Input: part model. Units: mm. Frame: model coordinates. A direction names the side the tool comes from. Coordinates: 2 decimals unless noted, no trailing zeros. Write each loop counter-clockwise with the first axis right and the second up, starting at its lowest first coordinate (ties: lowest second). Pieces come first, ordered by that corner, then holes. Notation, with made-up numbers: M -19,84 L 14,84 A32 ccw 14,114 Z; hole C 37,83.5 d9. An arc over 180 degrees is marked long. Write each question's results on one line, items separated by ' | '. Start each with the question number.
1. First-contact query: pin 1 (4.5 mm diameter, centred on x = 36.5, z = -2.5, fed in from +Y); pin 2 (1.5 mm diameter, centred on x = 38, z = 2.5, fed in from -Y); pin 3 (4 mm diameter, centred on y = 17.5, z = 2, fed in from -X). Flat tips, straight axial feed; report the tip coordinate or a pass-through.
2. Section query B-B, the plane z = -1.5. Output: boundary loops of the cut face in (x, y), and give its area (3 significant figures).
3. Set-up query: faces 5 (the flat face through (36, 20, -3)), 6 (the flat face through (38, 18.6, -2.5)), 7 (the cylindrical face through (17.94, 31.46, 4.81)). Return all of +Z, -Z, +X, -X, +Y, -Y with unobstructed straight access to the full face (end or side cutting, diameter ignored); none if empty.
4. Section query A-A, the plane x = -7. Output: boundary loops of the cut face in (y, z).
5. Section query C-C, the plane x = 1.5. Output: boundary loops of the cut face in (y, z).
6. Ray query, probe 1 along Y at (x, z) = (37.5, -2); probe 2 along Y at (x, z) = (-5, 0.75); probe 3 along X at (y, z) = (25, 3.5). Return the intervals inside material, ascending.
7. Section query D-D, the plane y = 5.5. Output: boundary loops of the cut face in (x, z).
8. Pull-direction query (Y, two-part tool) for faces 1 (the flat face through (10, 29, 2)), 2 (the flat face through (18.9, 30.2, 0.6)), 3 (the flat face through (39, 0, 2)), 4 (the flat face through (31, 15, 5)); classes: +Y half, -Y half, draft (parallel to the pull), parting line (faces both ways), or undercut.
```python
from build123d import *

# Parameters (mm, degrees)
SKETCH1_W           = 73
SKETCH1_H           = 29
BOSS_EXTRUDE1_DEPTH = 5
SKETCH2_R           = 1
CUT_EXTRUDE1_DEPTH  = 35
SKETCH3_W           = 4
SKETCH3_H           = 6
BOSS_EXTRUDE2_DEPTH = 5
SKETCH4_W           = 3
SKETCH4_H           = 2
CUT_EXTRUDE2_DEPTH  = 10
SKETCH5_R           = 2.5
BOSS_EXTRUDE3_DEPTH = 5
CUT_EXTRUDE3_DEPTH  = 25
FILLET1_R           = 1


with BuildPart() as part:
    # Sketch1 → Boss-Extrude1 (new body)
    with BuildSketch(Plane.XY):
        with Locations((36.5, 14.5)):
            Rectangle(SKETCH1_W, SKETCH1_H)
        Polygon((-10, 29), (0, 29), (5, 29), (5, 33), (-10, 33), align=None)
        Polygon((5, 0), (0, 0), (-10, 0), (-10, -4), (5, -4), align=None)
    extrude(amount=BOSS_EXTRUDE1_DEPTH)

    # Sketch2 → Cut-Extrude1 (cut)
    with BuildSketch(Plane(origin=(0, 33, 0), x_dir=(1, 0, 0), z_dir=(0, 1, 0))):
        with Locations(Location((-7, -2.46940408, 0), (0, 0, 270))):
            Circle(SKETCH2_R)
    extrude(amount=-CUT_EXTRUDE1_DEPTH, mode=Mode.SUBTRACT)

    # Sketch3 → Boss-Extrude2 (add)
    with BuildSketch(Plane(origin=(0, 0, 0), x_dir=(-1, 0, 0), z_dir=(0, 0, -1))):
        with Locations((-36, 20)):
            Rectangle(SKETCH3_W, SKETCH3_H)
    extrude(amount=BOSS_EXTRUDE2_DEPTH)

    # Sketch4 → Cut-Extrude2 (cut)
    with BuildSketch(Plane(origin=(38, 0, 0), x_dir=(0, 0, -1), z_dir=(1, 0, 0))):
        with Locations((1.5, 20)):
            Rectangle(SKETCH4_W, SKETCH4_H)
    extrude(amount=-CUT_EXTRUDE2_DEPTH, mode=Mode.SUBTRACT)

    # Sketch5 → Boss-Extrude3 (add)
    with BuildSketch(Plane(origin=(0, 29, 0), x_dir=(1, 0, 0), z_dir=(0, 1, 0))):
        with Locations(Location((18.894998898, -2.5, 0), (0, 0, 270))):
            Circle(SKETCH5_R)
    extrude(amount=BOSS_EXTRUDE3_DEPTH)

    # Sketch6 → Cut-Extrude3 (cut)
    with BuildSketch(Plane(origin=(5, 0, 0), x_dir=(0, 0, -1), z_dir=(1, 0, 0))):
        Polygon((0, 33), (-1, 31), (0, 29), align=None)
    extrude(amount=CUT_EXTRUDE3_DEPTH, mode=Mode.SUBTRACT)

    # Fillet1
    fillet1_edges = [part.edges().sort_by_distance(p)[0] for p in [
        (34, 20, -3),
        (38, 20, -3),
    ]]
    fillet(fillet1_edges, radius=FILLET1_R)


solid = part.part
```
Answer:
1) pin 1: y = 23 | pin 2: y = 0 | pin 3: x = 0
2) outline: M 34,17 L 38,17 L 38,19 L 34,19 Z; M 34,21 L 38,21 L 38,23 L 34,23 Z | area: 16.0 mm^2
3) face 5: +X, -X | face 6: -Z, +X, +Y, -Y | face 7: +Y
4) outline: M -4,0 L 0,0 L 0,1.47 L -2,1.47 L -2,3.47 L 0,3.47 L 0,5 L -4,5 Z; M 29,0 L 33,0 L 33,1.47 L 29,1.47 Z; M 29,3.47 L 33,3.47 L 33,5 L 29,5 Z
5) outline: M -4,0 L 33,0 L 33,5 L -4,5 Z
6) probe 1: 17 to 19, 21 to 23 | probe 2: -4 to 0, 29 to 33 | probe 3: 0 to 73
7) outline: M 0,0 L 73,0 L 73,5 L 0,5 Z
8) face 1: +Y half | face 2: undercut | face 3: -Y half | face 4: draft
